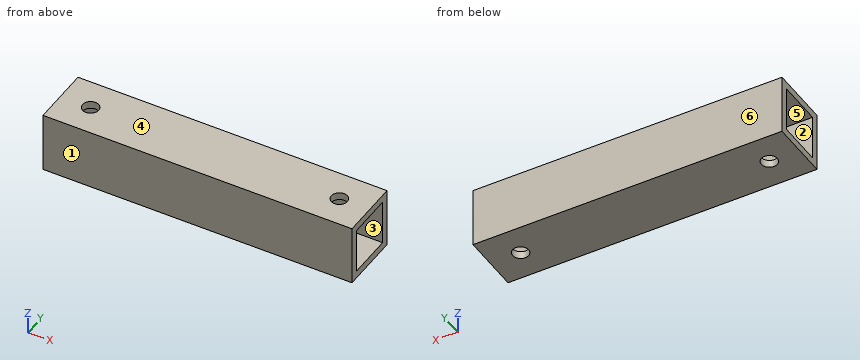
Autodesk Inventor part; units mm, degrees
ref_plane "YZ Plane" through (0, 0, 0) normal (1, 0, 0) x (0, 1, 0)
ref_plane "XZ Plane" through (0, 0, 0) normal (0, 1, 0) x (-1, 0, 0)
ref_plane "XY Plane" through (0, 0, 0) normal (0, 0, 1) x (1, 0, 0)
sketch "Sketch1" plane through (0, 0, 0) normal (1, 0, 0) x (0, 1, 0)
  line L0 (0, 0) -> (25.4, 0)
  line L1 (25.4, 0) -> (25.4, 25.4)
  line L2 (25.4, 25.4) -> (0, 25.4)
  line L3 (0, 25.4) -> (0, 0)
  line L4 (3.175, 22.225) -> (22.225, 22.225)
  line L5 (22.225, 22.225) -> (22.225, 3.175)
  line L6 (22.225, 3.175) -> (3.175, 3.175)
  line L7 (3.175, 3.175) -> (3.175, 22.225)
  dimension "d0" = 25.4
  dimension "d1" = 25.4
  dimension "d2" = 3.175
extrude "Extrusion1" add sketch "Sketch1" along normal blind 130.1496
sketch "Sketch2" plane through (0, 0, 0) normal (0, 0, -1) x (-1, 0, 0)
  circle A0 centre (-12.7, 12.7) radius 3.3734
  circle A1 centre (-117.4496, 12.7) radius 3.3734
  line L0 (0, 0) -> (0, 25.4)
  line L1 (-130.1496, 0) -> (-130.1496, 25.4)
  line L2 (0, 0) -> (-130.1496, 0)
  dimension "d5" = 6.7469
  dimension "d6" = 6.7469
  dimension "d7" = 12.7
  dimension "d8" = 12.7
  dimension "d9" = 12.7
  dimension "d10" = 12.7
extrude "Extrusion2" cut sketch "Sketch2" against normal blind 25.4
properties part number "support block"
Work out the finished part from the listing and answer in its coordinate system (mm). Face numbers are marked on the shaded views. A direction names the side the tool comes from. Give positions to 0.01 mm unless a question says otherwise; leave off trailing zeros. Loops run counter-clockwise (first coordinate to the right, second up) from the corner with the lowest first, then second, coordinate; pieces in that order, holes last. Notation, with made-up numbers: M 25.5,50.25 L 38.5,50.25 A20 cw 38.5,61.25 Z; hole C 60.5,45.25 d3. An arc over 180 degrees is marked long. One line per item, written item: value. Start each with the question number.
1. Find section B-B (y = 5.25). Give the vertices of the cut face in (x, z) (3 decimals).
2. Find section A-A (x = 12.7). Give the vertices of the cut face in (y, z) (3 decimals).
3. Determine the mould class of the marked faces 3, 4, 5 and 6 for opening direction Y: released by +Y, released by -Y, zero draft, split by the parting line, or undercut.
4. Find section C-C (x = 111.5). Give the vertices of the cut face in (y, z) (3 decimals), and give its area (3 significant figures).
5. Find the intervals of material crossed by probe 1 along Y at (x, z) = (65.5, 15.75) (3 decimals); probe 2 along X at (y, z) = (13, 3), in increasing order.
6. Which of the six approach directions +Z, -Z, +X, -X, +Y, -Y give full straight-line access (tool end or side, diameter ignored) to the marked faces 1 and 2?
Reported:
1. outline: M 0,0 L 130.15,0 L 130.15,3.175 L 0,3.175 Z; M 0,22.225 L 130.15,22.225 L 130.15,25.4 L 0,25.4 Z
2. outline: M 0,0 L 9.327,0 L 9.327,3.175 L 3.175,3.175 L 3.175,22.225 L 9.327,22.225 L 9.327,25.4 L 0,25.4 Z; M 16.073,0 L 25.4,0 L 25.4,25.4 L 16.073,25.4 L 16.073,22.225 L 22.225,22.225 L 22.225,3.175 L 16.073,3.175 Z
3. face 3: undercut
3. face 4: zero draft
3. face 5: undercut
3. face 6: released by +Y
4. outline: M 0,0 L 25.4,0 L 25.4,25.4 L 0,25.4 Z; hole M 3.175,3.175 L 22.225,3.175 L 22.225,22.225 L 3.175,22.225 Z
4. area: 282 mm²
5. probe 1: y = 0 to 3.175, 22.225 to 25.4
5. probe 2: x = 0 to 9.34, 16.06 to 114.09, 120.81 to 130.15
6. face 1: +Z, -Z, +X, -X, -Y
6. face 2: +X, -X
